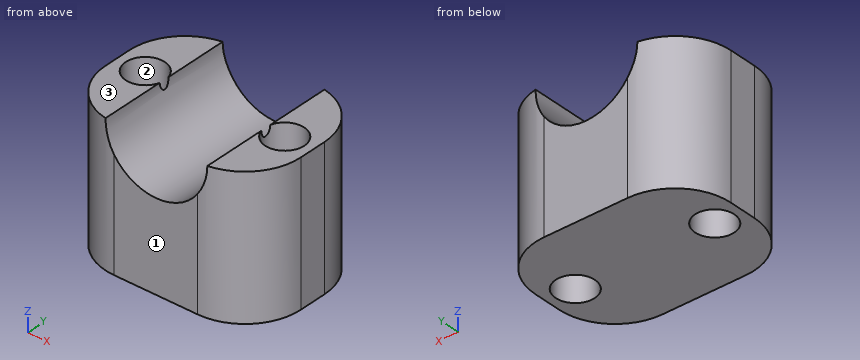
```python
from build123d import *

# Parameters (mm, degrees)
EXTRUDE_1_DEPTH     = 10
CUT_EXTRUDE_1_REACH = 17.78
SKETCH_2_R          = 3.65
CUT_EXTRUDE_2_REACH = 15.191
SKETCH_3_R          = 1.4


with BuildPart() as part:
    # Эскиз1 → Бобышка-Вытянуть1 (new body)
    with BuildSketch(Plane.XY):
        with BuildLine():
            Line((-3, 5), (3, 5))
            ThreePointArc((3, 5), (5.828427125, 3.828427125), (7, 1))
            Line((7, 1), (7, -1))
            ThreePointArc((7, -1), (5.828427125, -3.828427125), (3, -5))
            Line((3, -5), (-3, -5))
            ThreePointArc((-3, -5), (-5.828427125, -3.828427125), (-7, -1))
            Line((-7, -1), (-7, 1))
            ThreePointArc((-7, 1), (-5.828427125, 3.828427125), (-3, 5))
        make_face()
    extrude(amount=EXTRUDE_1_DEPTH)

    # Эскиз2 → Вырез-Вытянуть1 (cut, up to next)
    with BuildSketch(Plane(origin=(0, 5, 0), x_dir=(1, 0, 0), z_dir=(0, 1, 0)), mode=Mode.PRIVATE) as cut_extrude_1_sk1:
        with Locations((0, -10)):
            Circle(SKETCH_2_R)
    cut_extrude_1_tool1 = extrude(cut_extrude_1_sk1.sketch, amount=-CUT_EXTRUDE_1_REACH, mode=Mode.PRIVATE) & part.part
    add(cut_extrude_1_tool1.solids().sort_by_distance((0, 5, 10))[0], mode=Mode.SUBTRACT)

    # Эскиз3 → Вырез-Вытянуть2 (cut, up to next)
    with BuildSketch(Plane.XY.offset(10), mode=Mode.PRIVATE) as cut_extrude_2_sk1:
        with Locations((-5, 0)):
            Circle(SKETCH_3_R)
    cut_extrude_2_tool1 = extrude(cut_extrude_2_sk1.sketch, amount=-CUT_EXTRUDE_2_REACH, mode=Mode.PRIVATE) & part.part
    # Эскиз3 → Вырез-Вытянуть2 (cut, up to next)
    with BuildSketch(Plane.XY.offset(10), mode=Mode.PRIVATE) as cut_extrude_2_sk2:
        with Locations((5, 0)):
            Circle(SKETCH_3_R)
    cut_extrude_2_tool2 = extrude(cut_extrude_2_sk2.sketch, amount=-CUT_EXTRUDE_2_REACH, mode=Mode.PRIVATE) & part.part
    add(cut_extrude_2_tool1.solids().sort_by_distance((-5, 0, 10))[0], mode=Mode.SUBTRACT)
    add(cut_extrude_2_tool2.solids().sort_by_distance((5, 0, 10))[0], mode=Mode.SUBTRACT)


solid = part.part
```
CAD build for the part. Positions are in the model's coordinates, mm. Face numbers are marked on the shaded views. Coordinates: 2 decimals unless noted, no trailing zeros. Order: outer loops, then holes, each group sorted by start corner. A loop starts at its lowest first (then second) coordinate and runs counter-clockwise, first axis right, second up.
(1) Pin check, flat tips, straight feed: pin 1 Ø3 at (y, z) = (-4, 6.5) entering from +X; pin 2 Ø1.5 at (y, z) = (-3.5, 1.5) entering from -X. Stop position of each tip, or through.
Solution:
pin 1: stops at x = 6.71
pin 2: stops at x = -6.6
(2) Saw through at C-C, the plane x = 5. Write the cut outline in (y, z).
Solution:
outline: (-4.46, 0) - (-1.4, 0) - (-1.4, 10) - (-4.46, 10) - close; (1.4, 0) - (4.46, 0) - (4.46, 10) - (1.4, 10) - close
(3) Saw through at D-D, the plane z = 2.5. Write the cut outline in (x, y).
Solution:
outline: (-7, -1) arc R4 ccw to (-3, -5) - (3, -5) arc R4 ccw to (7, -1) - (7, 1) arc R4 ccw to (3, 5) - (-3, 5) arc R4 ccw to (-7, 1) - close; hole circle Ø2.8 at (-5, 0); hole circle Ø2.8 at (5, 0)
(4) Saw through at A-A, the plane z = 9. Write the cut outline in (x, y), and give its area (3 significant figures).
Solution:
outline: (-7, -1) arc R4 ccw to (-3.51, -4.97) - (-3.51, 4.97) arc R4 ccw to (-7, 1) - close; (3.51, -4.97) arc R4 ccw to (7, -1) - (7, 1) arc R4 ccw to (3.51, 4.97) - close; hole circle Ø2.8 at (-5, 0); hole circle Ø2.8 at (5, 0)
area: 43.8 mm2
(5) Drill centre lines: L1, parallel to X at y = -0.5, z = 8.75; L2, parallel to X at y = 0.75, z = 9.75; L3, parallel to Y at x = 4.5, z = 8.5. Where is each one in solid material? Low to high.
Solution:
L1: x = -7 to -6.31, -3.69 to -3.43, 3.43 to 3.69, 6.31 to 7
L2: x = -7 to -6.18, -3.82 to -3.64, 3.64 to 3.82, 6.18 to 7
L3: y = -4.71 to -1.31, 1.31 to 4.71
(6) Mould opens along Y. For the marked faces 1, 2 and 3 say: released by +Y, released by -Y, zero draft, split by the parting line, or undercut.
Solution:
face 1: released by -Y
face 2: undercut
face 3: zero draft
(7) Saw through at B-B, the plane y = 0. Write the cut outline in (x, z).
Solution:
outline: (-7, 0) - (-6.4, 0) - (-6.4, 10) - (-7, 10) - close; (-3.6, 0) - (3.6, 0) - (3.6, 9.4) arc R3.65 cw to (-3.6, 9.4) - close; (6.4, 0) - (7, 0) - (7, 10) - (6.4, 10) - close
